The listing builds one solid part. Answer for the finished solid, in the listing's coordinates (mm). A direction names the side the tool comes from. Give positions to 0.01 mm unless a question says otherwise; leave off trailing zeros. Loops run counter-clockwise (first coordinate to the right, second up) from the corner with the lowest first, then second, coordinate; pieces in that order, holes last. Notation, with made-up numbers: M 67.25,-24.75 L 103.25,-24.75 A24 cw 103.25,3.25 Z; hole C 28.5,77 d6. An arc over 180 degrees is marked long. Return JSON: item names as keys, results as strings.
from build123d import *

# Parameters (mm, degrees)
SKETCH_R     = 2
SKETCH_W     = 17.75
SKETCH_H     = 7.9
PAD_DEPTH    = 1.2
PAD001_DEPTH = 26
SKETCH002_W  = 5.95
SKETCH002_H  = 24.8
POCKET_DEPTH = 38.901
FILLET_R     = 1


with BuildPart() as part:
    # Sketch → Pad (new body)
    with BuildSketch(Plane.XY):
        with BuildLine():
            ThreePointArc((-13.5, 5.95), (-19.45, 0), (-13.5, -5.95))
            Line((-13.5, -5.95), (13.5, -5.95))
            ThreePointArc((13.5, -5.95), (19.45, 0), (13.5, 5.95))
            Line((-13.5, 5.95), (13.5, 5.95))
        make_face()
        with Locations((-13.5, 0)):
            Circle(SKETCH_R, mode=Mode.SUBTRACT)
        with Locations((13.5, 0)):
            Circle(SKETCH_R, mode=Mode.SUBTRACT)
        Rectangle(SKETCH_W, SKETCH_H, mode=Mode.SUBTRACT)
    extrude(amount=PAD_DEPTH)

    # Sketch001 (on Face12 of Pad) → Pad001 (join)
    with BuildSketch(Plane.XY.offset(1.2)):
        with BuildLine():
            Line((-19.45, 0), (-19.45, -39.95))
            Line((-19.45, -39.95), (19.45, -39.95))
            Line((19.45, -39.95), (19.45, 0))
            ThreePointArc((13.5, -5.95), (17.707285, -4.207285), (19.45, 0))
            Line((-13.5, -5.95), (13.5, -5.95))
            ThreePointArc((-19.45, 0), (-17.707285, -4.207285), (-13.5, -5.95))
        make_face()
    extrude(amount=-PAD001_DEPTH)

    # Sketch002 (on Face17 of Pad001) → Pocket (cut, through all)
    with BuildSketch(Plane.YZ.offset(19.45)):
        with Locations((-2.975, -12.4)):
            Rectangle(SKETCH002_W, SKETCH002_H)
        Polygon((-39.95, -3.2), (-37.55, -3.2), (-37.55, -0.8), (-8.45, -0.8), (-8.45, -22.8), (-37.55, -22.8), (-37.55, -20.4), (-39.95, -20.4), align=None)
    extrude(amount=-POCKET_DEPTH, mode=Mode.SUBTRACT)

    # Fillet
    fillet_edges = [part.edges().sort_by_distance(p)[0] for p in [
        (0, -8.45, -22.8),
        (0, -8.45, -0.8),
        (0, -37.55, -0.8),
        (0, -37.55, -3.2),
        (0, -39.95, -3.2),
        (0, -37.55, -20.4),
        (0, -39.95, -24.8),
        (0, -5.95, -24.8),
        (0, -39.95, -20.4),
        (0, -39.95, 1.2),
    ]]
    fillet(fillet_edges, radius=FILLET_R)


solid = part.part
(1) The part is cut by section C-C (x = 10). Determine the outline of the cut face in (y, z).
Values follow:
{"outline": "M -39.95,-23.8 A1 ccw -38.95,-24.8 L -6.95,-24.8 A1 ccw -5.95,-23.8 L -5.95,0 L 5.95,0 L 5.95,1.2 L -38.95,1.2 A1 ccw -39.95,0.2 L -39.95,-2.2 A1 ccw -38.95,-3.2 L -38.55,-3.2 A1 ccw -37.55,-2.2 L -37.55,-1.8 A1 cw -36.55,-0.8 L -9.45,-0.8 A1 cw -8.45,-1.8 L -8.45,-21.8 A1 cw -9.45,-22.8 L -37.55,-22.8 L -37.55,-21.4 A1 ccw -38.55,-20.4 L -38.95,-20.4 A1 ccw -39.95,-21.4 Z"}
(2) A tool of negligible diameter and unlimited length cuts with its end or side. For faces 4 (the cylindrical face through (-0.272, -8.751, -22.515)), 5 (the cylindrical face through (17.753, 4.161, 0.592)), 6 (the flat face through (0, -3.95, 1)), 7 (the flat face through (0, -5, 0)), 8 (the cylindrical face through (-0.272, -39.665, -20.701)), from which of +Z, -Z, +X, -X, +Y, -Y can it reach the whole face along a straight path? Write none if from no direction.
Values follow:
{"face 4": "+X, -X", "face 5": "+Z, -Z, +X, +Y", "face 6": "+Z, -Z", "face 7": "-Z, +X, -X, +Y", "face 8": "+X, -X, -Y"}
(3) The part is cut by section A-A (y = -23). Determine the outline of the cut face in (x, z).
Values follow:
{"outline": "M -19.45,-24.8 L 19.45,-24.8 L 19.45,-22.8 L -19.45,-22.8 Z; M -19.45,-0.8 L 19.45,-0.8 L 19.45,1.2 L -19.45,1.2 Z"}
(4) Given pin 1 (13 mm diameter, centred on x = 8.5, y = 2, fed in from -Z); pin 2 (1 mm diameter, centred on y = -29, z = -21.5, fed in from +X); pin 3 (2 mm diameter, centred on x = 0, z = -15, fed in from -Y); pin 4 (1.5 mm diameter, centred on x = -3.5, z = -22, fed in from +Y), each flat-ended and moving along its own axis, determine where each tip first touches the part or whether it passes through.
Values follow:
{"pin 1": "z = 0", "pin 2": "through", "pin 3": "y = -8.45", "pin 4": "y = -5.95"}
(5) The part is cut by section D-D (x = 14.5). Determine the outline of the cut face in (y, z), and give its area (3 significant figures).
Values follow:
{"outline": "M -39.95,-23.8 A1 ccw -38.95,-24.8 L -6.95,-24.8 A1 ccw -5.95,-23.8 L -5.95,0 L -1.73,0 L -1.73,1.2 L -38.95,1.2 A1 ccw -39.95,0.2 L -39.95,-2.2 A1 ccw -38.95,-3.2 L -38.55,-3.2 A1 ccw -37.55,-2.2 L -37.55,-1.8 A1 cw -36.55,-0.8 L -9.45,-0.8 A1 cw -8.45,-1.8 L -8.45,-21.8 A1 cw -9.45,-22.8 L -37.55,-22.8 L -37.55,-21.4 A1 ccw -38.55,-20.4 L -38.95,-20.4 A1 ccw -39.95,-21.4 Z; M 1.73,0 L 5.87,0 L 5.87,1.2 L 1.73,1.2 Z", "area": "212 mm²"}
(6) The part is cut by section B-B (x = 5.5). Determine the outline of the cut face in (y, z), and give its area (3 significant figures).
Values follow:
{"outline": "M -39.95,-23.8 A1 ccw -38.95,-24.8 L -6.95,-24.8 A1 ccw -5.95,-23.8 L -5.95,0 L -3.95,0 L -3.95,1.2 L -38.95,1.2 A1 ccw -39.95,0.2 L -39.95,-2.2 A1 ccw -38.95,-3.2 L -38.55,-3.2 A1 ccw -37.55,-2.2 L -37.55,-1.8 A1 cw -36.55,-0.8 L -9.45,-0.8 A1 cw -8.45,-1.8 L -8.45,-21.8 A1 cw -9.45,-22.8 L -37.55,-22.8 L -37.55,-21.4 A1 ccw -38.55,-20.4 L -38.95,-20.4 A1 ccw -39.95,-21.4 Z; M 3.95,0 L 5.95,0 L 5.95,1.2 L 3.95,1.2 Z", "area": "206 mm²"}
(7) Straight lines are drawn through the part: line 1 along Z through (x, y) = (14, -28); line 2 along Y through (x, z) = (-10.5, 0.25); line 3 along Z through (x, y) = (-8, -4.5). For each, find the intervals that lie inside material, in ascending order.
Values follow:
{"line 1": "-24.8 to -22.8, -0.8 to 1.2", "line 2": "-39.95 to 5.95", "line 3": "0 to 1.2"}
(8) Determine the mould class of faces 1 (the flat face through (0, -5.95, -12)), 2 (the flat face through (0, -23, -24.8)), 3 (the flat face through (0, -37.55, -22)) for opening direction Z: released by +Z, released by -Z, zero draft, split by the parting line, or undercut.
Values follow:
{"face 1": "zero draft", "face 2": "released by -Z", "face 3": "undercut"}
